Input: part model. Units: mm. Frame: model coordinates. Coordinates: 2 decimals unless noted, no trailing zeros. Write each loop counter-clockwise with the first axis right and the second up, starting at its lowest first coordinate (ties: lowest second). Pieces come first, ordered by that corner, then holes. Notation, with made-up numbers: (20.25, 49.5) - (67.25, 49.5) arc R31 cw to (67.25, 73.5) - close; hole circle Ø4 at (58, 73). An arc over 180 degrees is marked (long way). Use a Markdown table: item, result. Add a question column.
Q1. Section query D-D (x = 83.5). Return the cut outline in (y, z).
Q2. Section query A-A (x = 46). Return the cut outline in (y, z).
Q3. Section query C-C (z = 98). Return the cut outline in (x, y), then the cut area to 3 significant figures.
Q4. Mould query, pull axis Z, two halves, no side actions, for faces 1 (the face through (63, -63, 114.3)), 2 (the face through (63, -25.4, 84)), 3 (the face through (-1, -1, -63.5)). Classes: released by +Z, released by -Z, zero draft, split by the parting line, or undercut.
Q5. Material intervals for probe 1 along Z at (x, y) = (-34, 36.5); probe 2 along Y at (x, z) = (64.5, 96), sorted ascending. Write a range as from..to.
Q6. Section query B-B (y = -60). Return the cut outline in (x, z).
Q7. Pin query (flat end, axial travel): P1, Ø4, axis at y = 30, z = 43, coming from the +X side; P2, Ø23, axis at x = 69, y = -79.5, coming from the -Z side; P3, Ø6, axis at x = -40.5, z = -31.5, coming from the -Y side. Return the tip coordinate at first contact, or that it passes through.
from build123d import *

# Parameters (mm, degrees)
F0_W     = 127
F0_H     = 127
F1_DEPTH = 63.5
F4_DEPTH = 76.2
F5_W     = 38.1
F5_H     = 38.1
F6_DEPTH = 50.8


with BuildPart() as f1:
    # F0 (on Front) → F1 (new body, symmetric)
    with BuildSketch(Plane.XZ):
        Rectangle(F0_W, F0_H)
    extrude(amount=F1_DEPTH, both=True)

    # F3 (on offset) → F4 (join)
    with BuildSketch(Plane.XY.offset(38.1)):
        Polygon((101.6, -25.4), (63.5, -25.4), (63.5, -63.5), (25.4, -63.5), (25.4, -101.6), (101.6, -101.6), align=None)
    extrude(amount=F4_DEPTH)

    # F5 (on face) → F6 (join)
    with BuildSketch(Plane.XY.offset(63.5)):
        with Locations((44.45, -44.45)):
            Rectangle(F5_W, F5_H)
    extrude(amount=F6_DEPTH)


solid = f1.part
Values follow:
| question | item | result |
|---|---|---|
| 1 | outline | (-101.6, 38.1) - (-25.4, 38.1) - (-25.4, 114.3) - (-101.6, 114.3) - close |
| 2 | outline | (-101.6, 38.1) - (-63.5, 38.1) - (-63.5, -63.5) - (63.5, -63.5) - (63.5, 63.5) - (-25.4, 63.5) - (-25.4, 114.3) - (-101.6, 114.3) - close |
| 3 | outline | (25.4, -101.6) - (101.6, -101.6) - (101.6, -25.4) - (25.4, -25.4) - close |
| 3 | area | 5,810 mm2 |
| 4 | face 1 | released by +Z |
| 4 | face 2 | zero draft |
| 4 | face 3 | released by -Z |
| 5 | probe 1 | -63.5..63.5 |
| 5 | probe 2 | -101.6..-25.4 |
| 6 | outline | (-63.5, -63.5) - (63.5, -63.5) - (63.5, 38.1) - (101.6, 38.1) - (101.6, 114.3) - (25.4, 114.3) - (25.4, 63.5) - (-63.5, 63.5) - close |
| 7 | P1 | x = 63.5 |
| 7 | P2 | z = 38.1 |
| 7 | P3 | y = -63.5 |
